```python
from build123d import *

# Parameters (mm, degrees)
SKETCH_1_W          = 7
SKETCH_1_H          = 6
EXTRUDE_1_DEPTH     = 4
SKETCH_2_R          = 2
CUT_EXTRUDE_1_DEPTH = 11.049875621
EXTRUDE_2_REACH     = 12.05
SKETCH_7_R          = 1
CUT_EXTRUDE_3_DEPTH = 11.049875621


with BuildPart() as part:
    # 草图1 → 凸台-拉伸1 (new body)
    with BuildSketch(Plane.XY):
        with Locations((3.5, 3)):
            Rectangle(SKETCH_1_W, SKETCH_1_H)
    extrude(amount=EXTRUDE_1_DEPTH)

    # 草图2 → 切除-拉伸1 (cut, through all)
    with BuildSketch(Plane.ZY):
        with Locations((4, 3)):
            Circle(SKETCH_2_R)
    extrude(amount=-CUT_EXTRUDE_1_DEPTH, mode=Mode.SUBTRACT)

    # 草图6 → 凸台-拉伸2 (add, up to next)
    with BuildSketch(Plane.XY.offset(4), mode=Mode.PRIVATE) as extrude_2_sk1:
        Polygon((5.05, 5), (6, 5), (4.700321215, 1), (3.750321215, 1), align=None)
    extrude_2_tool1 = extrude(extrude_2_sk1.sketch, amount=-EXTRUDE_2_REACH, mode=Mode.PRIVATE) - part.part
    # 草图6 → 凸台-拉伸2 (add, up to next)
    with BuildSketch(Plane.XY.offset(4), mode=Mode.PRIVATE) as extrude_2_sk2:
        Polygon((2.1, 5), (3.05, 5), (1.750321215, 1), (0.800321215, 1), align=None)
    extrude_2_tool2 = extrude(extrude_2_sk2.sketch, amount=-EXTRUDE_2_REACH, mode=Mode.PRIVATE) - part.part
    add(extrude_2_tool1.solids().sort_by_distance((4.875161, 3, 4))[0])
    add(extrude_2_tool2.solids().sort_by_distance((1.925161, 3, 4))[0])

    # 草图7 → 切除-拉伸3 (cut, through all)
    with BuildSketch(Plane(origin=(7, 0, 0), x_dir=(0, 0, -1), z_dir=(1, 0, 0))):
        with Locations((-4, 3)):
            Circle(SKETCH_7_R)
    extrude(amount=-CUT_EXTRUDE_3_DEPTH, mode=Mode.SUBTRACT)


solid = part.part
```
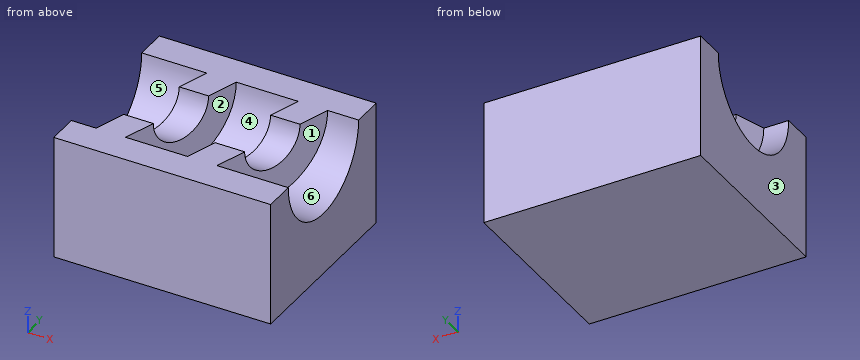
Check sheet for the modelled part. Datum: model origin and axes. Units: mm. Face numbers are marked on the shaded views. A direction names the side the tool comes from. Round coordinates to 2 decimals unless told otherwise and drop trailing zeros. Order: outer loops, then holes, each group sorted by start corner. A loop starts at its lowest first (then second) coordinate and runs counter-clockwise, first axis right, second up. Notation, with made-up numbers: (0.25, 83) -> (22.25, 83) arc R34 cw to (22.25, 115) -> close; hole circle Ø8 at (18, 11.25). An arc over 180 degrees is marked (long way). One line per item, written item: value. Start each with the question number.
Q1. Cross-section at D-D (z = 2.3). Record the boundary of the cut face in (x, y), and give its area (3 significant figures).
Q2. Cross-section at C-C (y = 3). Record the boundary of the cut face in (x, z).
Q3. Cross-section at B-B (x = 0.5). Record the boundary of the cut face in (y, z).
Q4. Thickness scan on line 1 (Y direction, x = 0.5, z = 2.7); line 2 (Y direction, x = 6.5, z = 2.45); line 3 (X direction, y = 2.1, z = 3.4). Record the ranges inside material, lowest first.
Q5. Mould release check, pull along X, two halves, no side actions. Record for the marked faces 1, 2 and 3: pulls with the +X half, pulls with the -X half, needs draft (parallel to the pull), parting line crosses it, or undercut.
Q6. Cross-section at A-A (z = 3.2). Record the boundary of the cut face in (x, y), and give its area (3 significant figures).
Q7. Gauge pin test, flat end, axial feed: pin 1 Ø1 at (y, z) = (2.5, 0.5) entering from -X. Record the tip position at first contact, or that the pin passes through.
Q8. Set-up check for the marked faces 4, 5 and 6: record each of +Z, -Z, +X, -X, +Y, -Y from which the full face is reachable in a straight line by a thin tool's end or side.
Completed:
1. outline: (0, 0) -> (7, 0) -> (7, 1.95) -> (5.01, 1.95) -> (5.69, 4.05) -> (7, 4.05) -> (7, 6) -> (0, 6) -> (0, 4.05) -> (1.79, 4.05) -> (1.11, 1.95) -> (0, 1.95) -> close; hole (2.06, 1.95) -> (4.06, 1.95) -> (4.74, 4.05) -> (2.74, 4.05) -> close
1. area: 31.3 mm²
2. outline: (0, 0) -> (7, 0) -> (7, 2) -> (5.35, 2) -> (5.35, 3) -> (4.4, 3) -> (4.4, 2) -> (2.4, 2) -> (2.4, 3) -> (1.45, 3) -> (1.45, 2) -> (0, 2) -> close
3. outline: (0, 0) -> (6, 0) -> (6, 4) -> (5, 4) arc R2 cw to (1, 4) -> (0, 4) -> close
4. line 1: y = 0 to 1.48, 4.52 to 6
4. line 2: y = 0 to 1.74, 4.26 to 6
4. line 3: x = 1.16 to 2.11, 4.11 to 5.06
5. face 1: pulls with the +X half
5. face 2: undercut
5. face 3: pulls with the -X half
6. outline: (0, 0) -> (7, 0) -> (7, 1.17) -> (4.75, 1.17) -> (5.16, 2.4) -> (4.21, 2.4) -> (3.8, 1.17) -> (1.8, 1.17) -> (2.21, 2.4) -> (1.26, 2.4) -> (0.85, 1.17) -> (0, 1.17) -> close; (0, 4.83) -> (2.05, 4.83) -> (1.65, 3.6) -> (2.6, 3.6) -> (3, 4.83) -> (5, 4.83) -> (4.6, 3.6) -> (5.55, 3.6) -> (5.95, 4.83) -> (7, 4.83) -> (7, 6) -> (0, 6) -> close
6. area: 21.0 mm²
7. pin 1: stops at x = 0
8. face 4: +Z
8. face 5: +Z, -X
8. face 6: +Z, +X
